Source: three-view drawing plus pictorial views. Frame: mm from the lowest corner of the part. A direction names the side the tool comes from. Coordinates: 2 decimals unless noted, no trailing zeros. Loops run counter-clockwise (first coordinate to the right, second up) from the corner with the lowest first, then second, coordinate; pieces in that order, holes last.
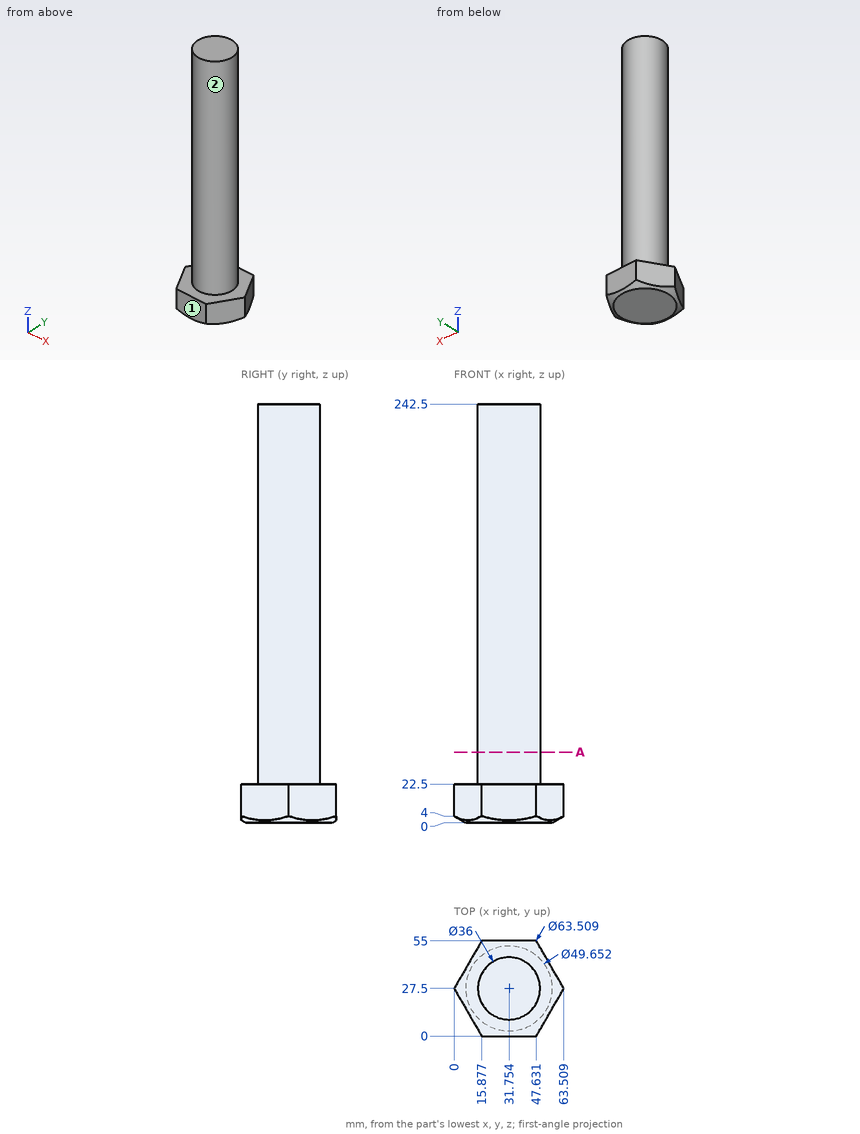
Q1. Line query: line 1 along Z through (x, y) = (48, 11); line 2 along Z through (x, y) = (52, 9); line 3 along Y through (x, z) = (21, 85) (1 decimal). Output: solid intervals per line, ascending.
Q2. Section A-A, the plane z = 41. Return the cut outline in (x, y) (1 decimal), plus the area to 3 significant figures.
Q3. Contact query for flat-ended pins moving along their axis: pin 1 Ø5 at (x, y) = (7, 9.5) entering from +Z; pin 2 Ø1 at (y, z) = (24.5, 169.5) entering from -X; pin 3 Ø6 at (y, z) = (33, 157) entering from +X; pin 4 Ø3 at (x, z) = (45, 138.5) entering from -Y. Output: stop coordinate, or through.
Q4. Access query for the marked faces 1 and 2. Directions: +Z, -Z, +X, -X, +Y, -Y. A direction counts if a zero-diameter tool reaches every point of the face in a straight line with its end or side. Return the directions, or none.
Derived:
1. line 1: z = 0 to 22.5
1. line 2: z = 1.5 to 22.5
1. line 3: y = 13.1 to 41.9
2. outline: circle Ø36 at (31.8, 27.5)
2. area: 1,020 mm2
3. pin 1: passes through
3. pin 2: stops at x = 13.93
3. pin 3: stops at x = 49.58
3. pin 4: stops at y = 13.86
4. face 1: +Z, -Z, +X, -X, -Y
4. face 2: +Z
